from build123d import *

# Parameters (mm, degrees)
SKETCH1_R           = 55
BOSS_EXTRUDE1_DEPTH = 26
SKETCH2_R           = 1.5
CUT_EXTRUDE1_DEPTH  = 3
SKETCH3_R           = 32.5
BOSS_EXTRUDE2_DEPTH = 8
SKETCH4_R           = 2.55
SKETCH4_R_2         = 1.55
SKETCH4_R_3         = 2.05
CUT_EXTRUDE2_DEPTH  = 3
FILLET1_R           = 2
SKETCH9_R           = 42.415927499
CUT_EXTRUDE3_DEPTH  = 83.012194282
SKETCH10_R          = 10
CUT_EXTRUDE4_DEPTH  = 5


with BuildPart() as part:
    # Sketch1 → Boss-Extrude1 (new body)
    with BuildSketch(Plane.XY):
        with Locations(Location((0, 0, 0), (0, 0, 180))):
            Circle(SKETCH1_R)
    extrude(amount=BOSS_EXTRUDE1_DEPTH)

    # Sketch2 → Cut-Extrude1 (cut)
    with BuildSketch(Plane(origin=(0, 0, 0), x_dir=(-1, 0, 0), z_dir=(0, 0, -1))):
        with Locations((0, -21)):
            Circle(SKETCH2_R)
        with Locations((-14.849242405, -14.849242405)):
            Circle(SKETCH2_R)
        with Locations((-21, 0)):
            Circle(SKETCH2_R)
        with Locations((-14.849242405, 14.849242405)):
            Circle(SKETCH2_R)
        with Locations((0, 21)):
            Circle(SKETCH2_R)
        with Locations((14.849242405, 14.849242405)):
            Circle(SKETCH2_R)
        with Locations((21, 0)):
            Circle(SKETCH2_R)
        with Locations((14.849242405, -14.849242405)):
            Circle(SKETCH2_R)
    extrude(amount=-CUT_EXTRUDE1_DEPTH, mode=Mode.SUBTRACT)

    # Sketch3 → Boss-Extrude2 (add)
    with BuildSketch(Plane.XY.offset(26)):
        Circle(SKETCH3_R)
    extrude(amount=BOSS_EXTRUDE2_DEPTH)

    # Sketch4 → Cut-Extrude2 (cut)
    with BuildSketch(Plane.XY.offset(34)):
        with Locations((-16.5, 0)):
            Circle(SKETCH4_R)
        with Locations((0, -16.5)):
            Circle(SKETCH4_R)
        with Locations((16.5, 0)):
            Circle(SKETCH4_R)
        with Locations((0, 16.5)):
            Circle(SKETCH4_R)
        with Locations((0, 26)):
            Circle(SKETCH4_R_2)
        with Locations((0, 22)):
            Circle(SKETCH4_R_2)
        with Locations((-11.66726189, -11.66726189)):
            Circle(SKETCH4_R_3)
        with Locations((11.66726189, -11.66726189)):
            Circle(SKETCH4_R_3)
        with Locations((11.66726189, 11.66726189)):
            Circle(SKETCH4_R_3)
        with Locations((-11.66726189, 11.66726189)):
            Circle(SKETCH4_R_3)
        with Locations((-22, 0)):
            Circle(SKETCH4_R_2)
        with Locations((-26, 0)):
            Circle(SKETCH4_R_2)
        with Locations((0, -22)):
            Circle(SKETCH4_R_2)
        with Locations((0, -26)):
            Circle(SKETCH4_R_2)
        with Locations((22, 0)):
            Circle(SKETCH4_R_2)
        with Locations((26, 0)):
            Circle(SKETCH4_R_2)
    extrude(amount=-CUT_EXTRUDE2_DEPTH, mode=Mode.SUBTRACT)

    # Fillet1
    fillet1_edges = [part.edges().sort_by_distance(p)[0] for p in [
        (55, 0, 0),
        (55, 0, 26),
    ]]
    fillet(fillet1_edges, radius=FILLET1_R)

    # Sketch9 → Cut-Extrude3 (cut, through all)
    with BuildSketch(Plane.XY.offset(26)):
        Circle(SKETCH9_R)
    extrude(amount=CUT_EXTRUDE3_DEPTH, mode=Mode.SUBTRACT)

    # Sketch10 → Cut-Extrude4 (cut)
    with BuildSketch(Plane.XY.offset(26)):
        Circle(SKETCH10_R)
    extrude(amount=-CUT_EXTRUDE4_DEPTH, mode=Mode.SUBTRACT)


solid = part.part
Source: CAD feature listing. Evaluate the final solid. Frame: model axes, mm. A direction names the side the tool comes from. Round coordinates to 2 decimals unless told otherwise and drop trailing zeros. Order: outer loops, then holes, each group sorted by start corner. A loop starts at its lowest first (then second) coordinate and runs counter-clockwise, first axis right, second up. Notation, with made-up numbers: (56, -21.75) - (66, -21.75) arc R17 cw to (66, -12.75) - close; hole circle Ø9 at (63, -37.75). An arc over 180 degrees is marked (long way). Use a Markdown table: item, result. Add a question column.
1. Section query B-B (z = 12.5). Return the cut outline in (x, y).
2. Section query A-A (y = 0). Return the cut outline in (x, z).
3. Line query: probe 1 along Y at (x, z) = (0, 22.6); probe 2 along Z at (x, y) = (-1, -1); probe 3 along Y at (x, z) = (-8.5, 7.75). Output: solid intervals per line, ascending.
4. Mould query, pull axis X, two halves, no side actions, for faces 1 (the cylindrical face through (-25.379, 48.794, 12.846)), 2 (the cylindrical face through (-14.524, -16.314, 1.479)), 3 (the flat face through (1, -1, 0)). Classes: +X half, -X half, draft (parallel to the pull), parting line (faces both ways), or undercut.
5. Set-up query: faces 4 (the cylindrical face through (-2.17, -9.76, 23.54)), 5 (the cylindrical face through (14.04, 16.11, 1.48)), 6 (the flat face through (-11, -1, 26)). Return all of +Z, -Z, +X, -X, +Y, -Y with unobstructed straight access to the full face (end or side cutting, diameter ignored); none if empty.
6. First-contact query: pin 1 (3.5 mm diameter, centred on x = 21.5, y = 0, fed in from -Z); pin 2 (1.5 mm diameter, centred on y = -32, z = 7, fed in from +X); pin 3 (0.9 mm diameter, centred on x = -14.5, y = 14.5, fed in from -Z); pin 4 (1.5 mm diameter, centred on x = 32.5, z = 16.5, fed in from -Y). Flat tips, straight axial feed; report the tip coordinate or a pass-through.
Derived:
| question | item | result |
|---|---|---|
| 1 | outline | circle Ø110 at (0, 0) |
| 2 | outline | (-55, 2) arc R2 ccw to (-53, 0) - (-22.5, 0) - (-22.5, 3) - (-19.5, 3) - (-19.5, 0) - (19.5, 0) - (19.5, 3) - (22.5, 3) - (22.5, 0) - (53, 0) arc R2 ccw to (55, 2) - (55, 24) arc R2 ccw to (53, 26) - (10, 26) - (10, 21) - (-10, 21) - (-10, 26) - (-53, 26) arc R2 ccw to (-55, 24) - close |
| 3 | probe 1 | -55 to -10, 10 to 55 |
| 3 | probe 2 | 0 to 21 |
| 3 | probe 3 | -54.34 to 54.34 |
| 4 | face 1 | parting line |
| 4 | face 2 | undercut |
| 4 | face 3 | draft |
| 5 | face 4 | +Z |
| 5 | face 5 | -Z |
| 5 | face 6 | +Z, +X, -X, +Y, -Y |
| 6 | pin 1 | z = 0 |
| 6 | pin 2 | x = 45.26 |
| 6 | pin 3 | z = 3 |
| 6 | pin 4 | y = -44.91 |
